from build123d import *

# Parameters (mm, degrees)
F1_DEPTH = 87
F3_W     = 30
F3_H     = 31.242104
F4_DEPTH = 25


with BuildPart() as f1:
    # F0 (on Front) → F1 (new body)
    with BuildSketch(Plane.XZ):
        Polygon((30, 40), (0, 40), (0, 0), (80, 0), (80, 20), (30, 20), align=None)
    extrude(amount=-F1_DEPTH)

    # F3 (on face) → F4 (join)
    with BuildSketch(Plane.XY.offset(40)):
        with Locations((0, 43.5)):
            Rectangle(F3_W, F3_H)
    extrude(amount=F4_DEPTH)


solid = f1.part
Work out the finished part from the listing and answer in its coordinate system (mm). A direction names the side the tool comes from. Give positions to 0.01 mm unless a question says otherwise; leave off trailing zeros. Write each loop counter-clockwise with the first axis right and the second up, starting at its lowest first coordinate (ties: lowest second). Pieces come first, ordered by that corner, then holes. Notation, with made-up numbers: M 16,61 L 46,61 A27 cw 46,96 Z; hole C 8.25,3 d3. An arc over 180 degrees is marked long. Answer as CSV lines item,"result".
Q1. A cutting plane is placed at D-D on y = 81.5. Write down the section's boundary in (x, z).
A:
outline,"M 0,0 L 80,0 L 80,20 L 30,20 L 30,40 L 0,40 Z"
Q2. A cutting plane is placed at B-B on x = 1.5. Write down the section's boundary in (y, z).
A:
outline,"M 0,0 L 87,0 L 87,40 L 59.12,40 L 59.12,65 L 27.88,65 L 27.88,40 L 0,40 Z"
Q3. A cutting plane is placed at C-C on z = 16.5. Write down the section's boundary in (x, y).
A:
outline,"M 0,0 L 80,0 L 80,87 L 0,87 Z"
Q4. A cutting plane is placed at A-A on y = 35. Write down the section's boundary in (x, z).
A:
outline,"M -15,40 L 0,40 L 0,0 L 80,0 L 80,20 L 30,20 L 30,40 L 15,40 L 15,65 L -15,65 Z"
Q5. Given P1, Ø12, axis at y = 60, z = 24, coming from the -X side; P2, Ø1.5, axis at y = 73.5, z = 40.5, coming from the +X side; P3, Ø7.5, axis at x = -9, y = 42, coming from the -Z side, each flat-ended and moving along its own axis, determine where each tip first touches the part or whether it passes through.
A:
P1,"stops at x = 0"
P2,"stops at x = 30"
P3,"stops at z = 40"
Q6. Find the intervals of material crossed by probe 1 along X at (y, z) = (79, 35.5); probe 2 along X at (y, z) = (40.5, 50.5); probe 3 along Y at (x, z) = (-3, 49), in increasing order. Write a range as [from, to].
A:
probe 1,"x = [0, 30]"
probe 2,"x = [-15, 15]"
probe 3,"y = [27.88, 59.12]"
Q7. A tool of negligible diameter and unlimited length cuts with its end or side. For faces 1 (the flat face through (0, 59.121, 52)), 2 (the flat face through (0, 27.879, 52)), 3 (the flat face through (15, 43, 52)), 4 (the flat face through (0, 43, 20)), from which of +Z, -Z, +X, -X, +Y, -Y can it reach the whole face along a straight path? Write none if from no direction.
A:
face 1,"+Z, +X, -X, +Y"
face 2,"+Z, +X, -X, -Y"
face 3,"+Z, +X, +Y, -Y"
face 4,"-Z, -X, +Y, -Y"
